Autodesk Inventor part; units mm, degrees
ref_plane "YZ Plane" through (0, 0, 0) normal (1, 0, 0) x (0, 1, 0)
ref_plane "XZ Plane" through (0, 0, 0) normal (0, 1, 0) x (-1, 0, 0)
ref_plane "XY Plane" through (0, 0, 0) normal (0, 0, 1) x (1, 0, 0)
sketch "Sketch1" plane through (0, 0, 0) normal (0, 0, 1) x (1, 0, 0)
  arc A0 (31.877, -6.35) -> (-31.877, -6.35) centre (0, -83.1863) ccw
  line L0 (-31.877, -6.35) -> (31.877, -6.35) construction
  line L1 (0, 36.3731) -> (0, -103.1128) construction
  line L2 (-44.6278, 0) -> (44.6278, 0) construction
  line L3 (-31.877, -6.35) -> (-31.877, -4.497)
  line L4 (-31.877, 16.4465) -> (31.877, 16.4465)
  line L5 (31.877, 16.4465) -> (31.877, -2.4453)
  line L6 (-30.1625, 16.4465) -> (-30.1625, 5.334) construction
  line L7 (-30.1625, 5.334) -> (30.1625, 5.334) construction
  line L8 (30.1625, 5.334) -> (30.1625, 16.4465) construction
  arc A1 (31.877, -4.497) -> (-31.877, -4.497) centre (0, -83.1863) ccw
  arc A2 (31.877, -2.4453) -> (-31.877, -2.4453) centre (0, -83.1863) ccw
  line L9 (-30.1625, 13.1134) -> (-26.9875, 13.1134) construction
  line L10 (-26.9875, 13.1134) -> (-26.9875, 5.334) construction
  line L11 (30.1625, 12.4907) -> (26.9875, 12.4907) construction
  line L12 (26.9875, 12.4907) -> (26.9875, 5.334) construction
  line L13 (-31.877, -2.4453) -> (-31.877, 16.4465)
  line L14 (-31.877, -4.497) -> (-31.877, -2.4453)
  line L15 (31.877, -2.4453) -> (31.877, -4.497)
  line L16 (31.877, -4.497) -> (31.877, -6.35)
  point P0 (0, 0)
  point P1 (0, 3.6195)
  dimension "d0" = 1.7145
  dimension "d2" = 1.7145
  dimension "d3" = 1.905
  dimension "d4" = 1.7145
  dimension "d5" = 1.7145
  dimension "d6" = 11.1125
  dimension "d7" = 3.175
  dimension "d8" = 3.175
  dimension "d10" = 60.325
  dimension "d11" = 6.35
extrude "Extrusion1" add sketch "Sketch1" along normal mid plane 63.754
sketch "Sketch2" plane through (-31.877, 16.4465, 31.877) normal (0, 1, 0) x (1, 0, 0)
  line L0 (62.0395, 1.7145) -> (1.7145, 1.7145)
  line L1 (1.7145, 1.7145) -> (1.7145, 11.684)
  line L2 (1.7145, 62.0395) -> (62.0395, 62.0395)
  line L3 (62.0395, 62.0395) -> (62.0395, 52.07)
  line L4 (62.0395, 1.7145) -> (1.7145, 62.0395) construction
  line L5 (1.7145, 1.7145) -> (62.0395, 62.0395) construction
  line L6 (0, 63.754) -> (0, 0)
  line L7 (76.5048, 31.877) -> (-12.7508, 31.877) construction
  line L8 (31.877, 76.5048) -> (31.877, -12.7508) construction
  line L9 (1.7145, 11.684) -> (62.0395, 11.684)
  line L10 (1.7145, 11.684) -> (1.7145, 52.07)
  line L11 (1.7145, 52.07) -> (62.0395, 52.07)
  line L12 (1.7145, 52.07) -> (1.7145, 62.0395)
  line L13 (62.0395, 11.684) -> (62.0395, 1.7145)
  line L14 (0, 63.754) -> (63.754, 63.754)
  line L15 (4.8895, 50.8) -> (63.754, 50.8)
  line L16 (4.8895, 50.8) -> (4.8895, 12.954)
  line L17 (63.754, 63.754) -> (63.754, 0)
  line L18 (63.754, 50.8) -> (63.754, 12.954)
  line L19 (63.754, 0) -> (63.754, 63.754)
  line L20 (4.8895, 12.954) -> (63.754, 12.954)
  line L21 (62.0395, 11.684) -> (63.754, 11.684)
  line L22 (63.754, 12.954) -> (63.754, 11.684)
  line L23 (62.0395, 52.07) -> (63.754, 52.07)
  line L24 (63.754, 52.07) -> (63.754, 50.8)
  point P0 (31.877, 31.877)
  dimension "d14" = 1.7145
  dimension "d17" = 1.7145
  dimension "d34" = 1.27
  dimension "d35" = 1.7145
  dimension "d36" = 3.175
  dimension "d37" = 40.386
extrude "Extrusion2" cut sketch "Sketch2" against normal blind 11.1125 contours L20 L16 L15 L17
extrude "Extrusion3" cut sketch "Sketch2" against normal blind 1.778 contours L9 L10 L11 L23 L17 L15 L16 L20 L21
extrude "Extrusion6" cut sketch "Sketch1" along normal mid plane 26.035 contours A1 L14 A2 L15
fillet "Fillet1" radius 9.525 4 edges at (31.877, 5.0483, 31.877) (31.877, 5.0483, -31.877) (-31.877, 5.0483, 31.877) (-31.877, 5.0483, -31.877)
sketch "Sketch6" plane through (-26.9875, 5.334, 18.923) normal (1, 0, 0) x (0, 0, -1)
  circle A0 centre (18.923, 4.6673) radius 3.81
  circle A1 centre (18.923, 4.6673) radius 2.8575
  line L0 (0, 0) -> (0, 9.3345)
  line L1 (37.846, 0) -> (0, 0)
  point P0 (18.923, -5.334)
  point P1 (0, 4.6673)
  point P2 (18.923, 0)
  dimension "d38" = 7.62
  dimension "d39" = 5.715
extrude "Extrusion7" cut sketch "Sketch6" against normal up to next contours A1
extrude "Extrusion8" cut sketch "Sketch6" against normal blind 3.175
sketch "Sketch7" plane through (-30.1625, 16.4465, 20.193) normal (0, 1, 0) x (1, 0, 0)
  line L0 (7.8105, 52.07) -> (52.5145, 52.07)
  arc A0 (7.8105, 52.07) -> (-1.7145, 42.545) centre (7.8105, 42.545) ccw
  arc A1 (62.0395, 42.545) -> (52.5145, 52.07) centre (52.5145, 42.545) ccw
  line L1 (-1.7145, -2.159) -> (-1.7145, 42.545)
  arc A2 (-1.7145, -2.159) -> (7.8105, -11.684) centre (7.8105, -2.159) ccw
  line L2 (52.5145, -11.684) -> (7.8105, -11.684)
  arc A3 (52.5145, -11.684) -> (62.0395, -2.159) centre (52.5145, -2.159) ccw
  line L3 (62.0395, 42.545) -> (62.0395, 40.386)
  line L4 (62.0395, 42.545) -> (62.0395, 39.116)
  line L5 (62.0395, 39.116) -> (3.175, 39.116)
  line L6 (3.175, 39.116) -> (3.175, 1.27)
  line L7 (3.175, 1.27) -> (62.0395, 1.27)
  line L8 (62.0395, 39.116) -> (62.0395, 1.27)
  line L9 (62.0395, 1.27) -> (62.0395, -2.159)
  point P0 (30.1625, 20.193)
extrude "Extrusion9" add sketch "Sketch7" along normal blind 1.778 contours L0 A1 L3 L4 L5 L6 L7 L9 A3 L2 A2 L1 A0
sketch "Sketch8" plane through (-30.1625, 18.2245, 20.193) normal (0, 1, 0) x (1, 0, 0)
  line L0 (52.5145, 52.07) -> (7.8105, 52.07)
  arc A0 (62.0395, 42.545) -> (52.5145, 52.07) centre (52.5145, 42.545) ccw
  arc A1 (7.8105, 52.07) -> (-1.7145, 42.545) centre (7.8105, 42.545) ccw
  line L1 (-1.7145, 42.545) -> (-1.7145, -2.159)
  arc A2 (-1.7145, -2.159) -> (7.8105, -11.684) centre (7.8105, -2.159) ccw
  line L2 (7.8105, -11.684) -> (52.5145, -11.684)
  arc A3 (52.5145, -11.684) -> (62.0395, -2.159) centre (52.5145, -2.159) ccw
  line L3 (62.0395, -2.159) -> (62.0395, 42.545)
  line L4 (62.0395, 42.545) -> (62.0395, -2.159)
  circle A4 centre (30.1625, 20.193) radius 27.94
  dimension "d47" = 55.88
extrude "Extrusion10" add sketch "Sketch8" along normal blind 6.35
fillet "Fillet2" radius 3.175 8 edges at (29.0872, 24.5745, 29.0872) (31.877, 24.5745, 0) (29.0872, 24.5745, -29.0872) (0, 24.5745, -31.877) (-29.0872, 24.5745, -29.0872) (-31.877, 24.5745, 0) (-29.0872, 24.5745, 29.0872) (0, 24.5745, 31.877)
equation "\"d17\" = d14"
equation "\"d35\" = d17"
equation "\"d18\" = d6"
properties part number "Track v3"
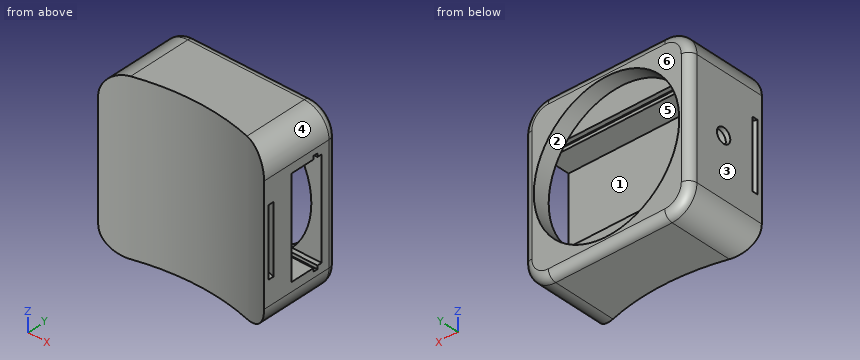
Source: CAD feature listing. Evaluate the final solid. Frame: model axes, mm. Face numbers are marked on the shaded views. A direction names the side the tool comes from. Give positions to 0.01 mm unless a question says otherwise; leave off trailing zeros. Use a Markdown table: item, result. Add a question column.
1) Reachability of the marked faces 1, 2 and 3 from +Z, -Z, +X, -X, +Y, -Y: full face, straight path, thin tool, end or side. Return the list, or none.
2) Section query A-A, the plane z = 0. Count the separate pieces of the cut face and the enclosed holes in it, then the cut area to 3 significant figures.
3) Line query: line 1 along Y through (x, z) = (-27.55, 0); line 2 along X through (y, z) = (21, 0); line 3 along Z through (x, y) = (1, 15). Output: solid intervals per line, ascending. Write a range as [from, to].
4) Pull-direction query (Y, two-part tool) for the marked faces 4, 5 and 6; classes: +Y half, -Y half, draft (parallel to the pull), parting line (faces both ways), or undercut.
5) First-contact query: pin 1 (4.5 mm diameter, centred on x = -10, z = -23.5, fed in from +Y); pin 2 (0.5 mm diameter, centred on y = 15.5, z = 1, fed in from +X); pin 3 (1.5 mm diameter, centred on x = 20, z = 21, fed in from -Y); pin 4 (3.5 mm diameter, centred on y = 10, z = 0, fed in from +X). Flat tips, straight axial feed; report the tip coordinate or a pass-through.
Numbers:
| question | item | result |
|---|---|---|
| 1 | face 1 | +X |
| 1 | face 2 | +Y |
| 1 | face 3 | +Z, -Z, -X, +Y, -Y |
| 2 | separate pieces | 4 |
| 2 | enclosed holes | 0 |
| 2 | area | 418 mm2 |
| 3 | line 1 | y = [-4.69, -2.88], [-0.87, 6.19], [13.81, 14.67], [16.45, 18.22] |
| 3 | line 2 | x = [-31.88, -27.94], [27.94, 31.88] |
| 3 | line 3 | z = [-31.88, -20.19], [20.19, 31.88] |
| 4 | face 4 | draft |
| 4 | face 5 | undercut |
| 4 | face 6 | +Y half |
| 5 | pin 1 | stops at y = 18.22 |
| 5 | pin 2 | stops at x = -30.16 |
| 5 | pin 3 | stops at y = -2.63 |
| 5 | pin 4 | passes through |
